Part model, mm, in its own coordinate system. Coordinates: 2 decimals unless noted, no trailing zeros. Order: outer loops, then holes, each group sorted by start corner. A loop starts at its lowest first (then second) coordinate and runs counter-clockwise, first axis right, second up.
from build123d import *

# Parameters (mm, degrees)
SKETCH1_W           = 76.2
SKETCH1_H           = 254
BOSS_EXTRUDE1_DEPTH = 3.175
SKETCH2_W           = 3.175
SKETCH2_H           = 254
BOSS_EXTRUDE2_DEPTH = 25.4
BOSS_EXTRUDE3_REACH = 75.025
SKETCH3_W           = 254
SKETCH3_H           = 3.175
SKETCH4_R           = 3.3782
CUT_EXTRUDE1_DEPTH  = 29.575
SKETCH5_R           = 3
CUT_EXTRUDE2_DEPTH  = 29.575


with BuildPart() as part:
    # Sketch1 → Boss-Extrude1 (new body)
    with BuildSketch(Plane(origin=(0, 0, 0), x_dir=(1, 0, 0), z_dir=(0, 1, 0))):
        with Locations((38.1, 127)):
            Rectangle(SKETCH1_W, SKETCH1_H)
    extrude(amount=BOSS_EXTRUDE1_DEPTH)

    # Sketch2 → Boss-Extrude2 (add)
    with BuildSketch(Plane(origin=(0, 3.175, 0), x_dir=(1, 0, 0), z_dir=(0, 1, 0))):
        with Locations((1.5875, 127)):
            Rectangle(SKETCH2_W, SKETCH2_H)
        with Locations((74.6125, 127)):
            Rectangle(SKETCH2_W, SKETCH2_H)
    extrude(amount=BOSS_EXTRUDE2_DEPTH)

    # Sketch3 → Boss-Extrude3 (add, up to next)
    with BuildSketch(Plane(origin=(3.175, 0, 0), x_dir=(0, 0, -1), z_dir=(1, 0, 0)), mode=Mode.PRIVATE) as boss_extrude3_sk1:
        with Locations((127, 26.9875)):
            Rectangle(SKETCH3_W, SKETCH3_H)
    boss_extrude3_tool1 = extrude(boss_extrude3_sk1.sketch, amount=BOSS_EXTRUDE3_REACH, mode=Mode.PRIVATE) - part.part
    add(boss_extrude3_tool1.solids().sort_by_distance((3.175, 26.9875, -127))[0])

    # Sketch4 → Cut-Extrude1 (cut, through all)
    with BuildSketch(Plane.XZ):
        with Locations((34.5313, -191.01308)):
            Circle(SKETCH4_R)
        with Locations((34.5313, -207.60436)):
            Circle(SKETCH4_R)
        with Locations((34.5313, -224.19564)):
            Circle(SKETCH4_R)
        with Locations((34.5313, -240.78692)):
            Circle(SKETCH4_R)
    extrude(amount=-CUT_EXTRUDE1_DEPTH, mode=Mode.SUBTRACT)

    # Sketch5 → Cut-Extrude2 (cut, through all)
    with BuildSketch(Plane(origin=(0, 28.575, 0), x_dir=(1, 0, 0), z_dir=(0, 1, 0))):
        with Locations((14.2875, 10.852567875)):
            Circle(SKETCH5_R)
        with Locations((61.9125, 10.852567875)):
            Circle(SKETCH5_R)
    extrude(amount=-CUT_EXTRUDE2_DEPTH, mode=Mode.SUBTRACT)


solid = part.part
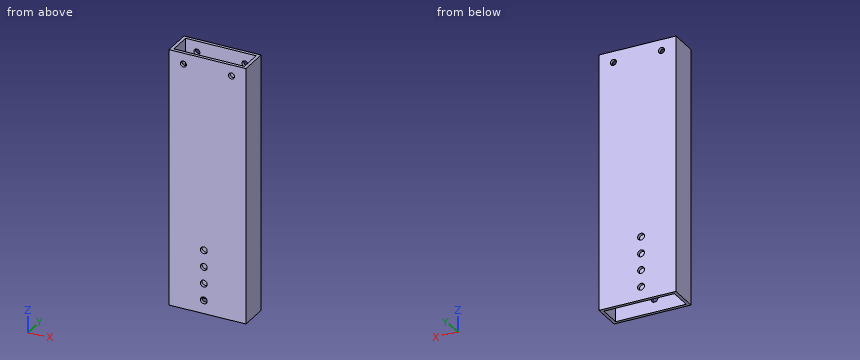
Q1. Cut at C-C on z = -149. Write the cut outline in (x, y) (3 decimals).
Results list:
outline: (0, 0) - (76.2, 0) - (76.2, 28.575) - (0, 28.575) - close; hole (3.175, 3.175) - (73.025, 3.175) - (73.025, 25.4) - (3.175, 25.4) - close
Q2. Cut at D-D on x = 33.5. Count the separate pieces of the cut face and the enclosed holes in it, and give its area (3 significant figures).
Results list:
separate pieces: 10
enclosed holes: 0
area: 1,450 mm2
Q3. Cut at B-B on y = 15. Write the cut outline in (x, z) (3 decimals), and give its area (3 significant figures).
Results list:
outline: (0, -254) - (3.175, -254) - (3.175, 0) - (0, 0) - close; (73.025, -254) - (76.2, -254) - (76.2, 0) - (73.025, 0) - close
area: 1,610 mm2
Q4. Cut at A-A on x = 20.5. Write the cut outline in (y, z) (3 decimals), and give its area (3 significant figures).
Results list:
outline: (0, -254) - (3.175, -254) - (3.175, 0) - (0, 0) - close; (25.4, -254) - (28.575, -254) - (28.575, 0) - (25.4, 0) - close
area: 1,610 mm2
Q5. Wall check: line 1 along X through (y, z) = (23.25, -24.5) (3 decimals); line 2 along Y through (x, z) = (72.5, -191.5) (3 decimals); line 3 along X through (y, z) = (27, -190). Give the ranges that are in metal, low to high.
Results list:
line 1: x = 0 to 3.175, 73.025 to 76.2
line 2: y = 0 to 3.175, 25.4 to 28.575
line 3: x = 0 to 31.31, 37.75 to 76.2
Q6. Pin check, flat tip, straight feed: pin 1 Ø6 at (x, z) = (34.53, -207.6) entering from +Y. Stop position of the tip, or through.
Results list:
pin 1: passes through
